Solid Edge part; units mm, degrees
sketch "Sketch1" plane through (0, 0, 0) normal (0, 0, 1) x (1, 0, 0)
  arc A0 (-1.8, 0) -> (-1.0449, 2.0645) centre (1.4, 0) cw
  arc A1 (-1.0449, 2.0645) -> (-0.9685, 2.1) centre (-0.9685, 2) cw
  line L0 (-0.9685, 2.1) -> (0, 2.1)
  line L1 (0, 2.1) -> (0, 1.2)
  arc A2 (0, 1.2) -> (0.1, 1.1) centre (0.1, 1.2) ccw
  line L2 (0.1, 1.1) -> (4.5, 1.1)
  line L3 (4.5, 1.1) -> (6.5, 0)
  line L4 (6.5, 0) -> (-1.8, 0)
revolve "RevolvedProtrusion1" add sketch "Sketch1" angle 360 about axis through (9.5, 0, 0) along (-1, 0, 0)
cosmetic_thread "Thread1"
sketch "Sketch2" plane through (0, 0, 0) normal (0, 0, 1) x (1, 0, 0)
  line L0 (-1.8, -1) -> (-1.2, -1)
  line L1 (-1.2, -1) -> (-0.6, -0.4)
  line L2 (-0.6, -0.4) -> (-0.6, 0.4)
  line L3 (-0.6, 0.4) -> (-1.2, 1)
  line L4 (-1.2, 1) -> (-1.8, 1)
  line L5 (-1.8, 1) -> (-1.8, -1)
extrude "ExtrudedCutout_1" cut sketch "Sketch2" against normal blind 0.25 and the other way blind 0.25
sketch "Sketch3" plane through (0, 0, 0) normal (0, -1, 0) x (1, 0, 0)
  line L0 (-1.9, 1) -> (-1.21, 1)
  line L1 (-1.21, 1) -> (-0.61, 0.4)
  line L2 (-0.61, 0.4) -> (-0.61, -0.4)
  line L3 (-0.61, -0.4) -> (-1.21, -1)
  line L4 (-1.21, -1) -> (-1.9, -1)
  line L5 (-1.9, -1) -> (-1.9, 1)
extrude "ExtrudedCutout_2" cut sketch "Sketch3" against normal blind 0.25 and the other way blind 0.25
sketch "Sketch4" plane through (-0.8, 0, 0) normal (1, 0, 0) x (0, 1, 0)
  line L0 (-0.7071, 0.7071) -> (-0.1138, 0)
  line L1 (-0.1138, 0) -> (-0.7071, -0.7071)
  line L2 (-0.7071, -0.7071) -> (0, -0.1138)
  line L3 (0, -0.1138) -> (0.7071, -0.7071)
  line L4 (0.7071, -0.7071) -> (0.1138, 0)
  line L5 (0.1138, 0) -> (0.7071, 0.7071)
  line L6 (0.7071, 0.7071) -> (0, 0.1138)
  line L7 (0, 0.1138) -> (-0.7071, 0.7071)
extrude "ExtrudedCutout_3" cut sketch "Sketch4" against normal blind 1.8
properties part number "bene_inox_412405-2,2X6,5"
Geometry: final body of the model. Coordinates: model frame, mm. A direction names the side the tool comes from. Coordinates: 2 decimals unless noted, no trailing zeros. Order: outer loops, then holes, each group sorted by start corner. A loop starts at its lowest first (then second) coordinate and runs counter-clockwise, first axis right, second up. Notation, with made-up numbers: M -8,75.25 L 11,75.25 A29 ccw 11,110.25 Z; hole C 19,-35.5 d2. An arc over 180 degrees is marked long. One line per question, with ' | ' between items. Start each with the question number.
Item 1: Set-up query: faces 1 (the cylindrical face through (-0.477, 2.003, 0.631)), 2 (the flat face through (0, 1, 1)). Return all of +Z, -Z, +X, -X, +Y, -Y with unobstructed straight access to the full face (end or side cutting, diameter ignored); none if empty.
Item 2: Ray query, probe 1 along Y at (x, z) = (-0.75, 0.4); probe 2 along X at (y, z) = (0.8, -1.9); probe 3 along X at (y, z) = (-0.35, -1.9). Return the intervals inside material, ascending. Write a range as [from, to].
Item 3: Cut plane B-B, the plane x = 0.75. Return the cut outline in (y, z), then the cut area to 3 significant figures.
Item 4: Cut plane A-A, the plane x = 5.5. Return the cut outline in (y, z), then the cut area to 3 significant figures.
Item 5: Pin query (flat end, axial travel): pin 1 Ø0.5 at (y, z) = (-0.5, -0.5) entering from -X; pin 2 Ø0.6 at (x, z) = (-1, 0.5) entering from +Y; pin 3 Ø0.8 at (x, z) = (-1, -1) entering from -Y. Return the tip coordinate at first contact, or that it passes through.
A:
1) face 1: +X, -X | face 2: +X
2) probe 1: y = [-2.06, -0.25], [0.25, 2.06] | probe 2: x = [-1.05, 0] | probe 3: x = [-1.15, 0]
3) outline: C 0,0 d2.2 | area: 3.80 mm2
4) outline: C 0,0 d1.1 | area: 0.950 mm2
5) pin 1: stops at x = -1.77 | pin 2: stops at y = 2.09 | pin 3: stops at y = -2.01
